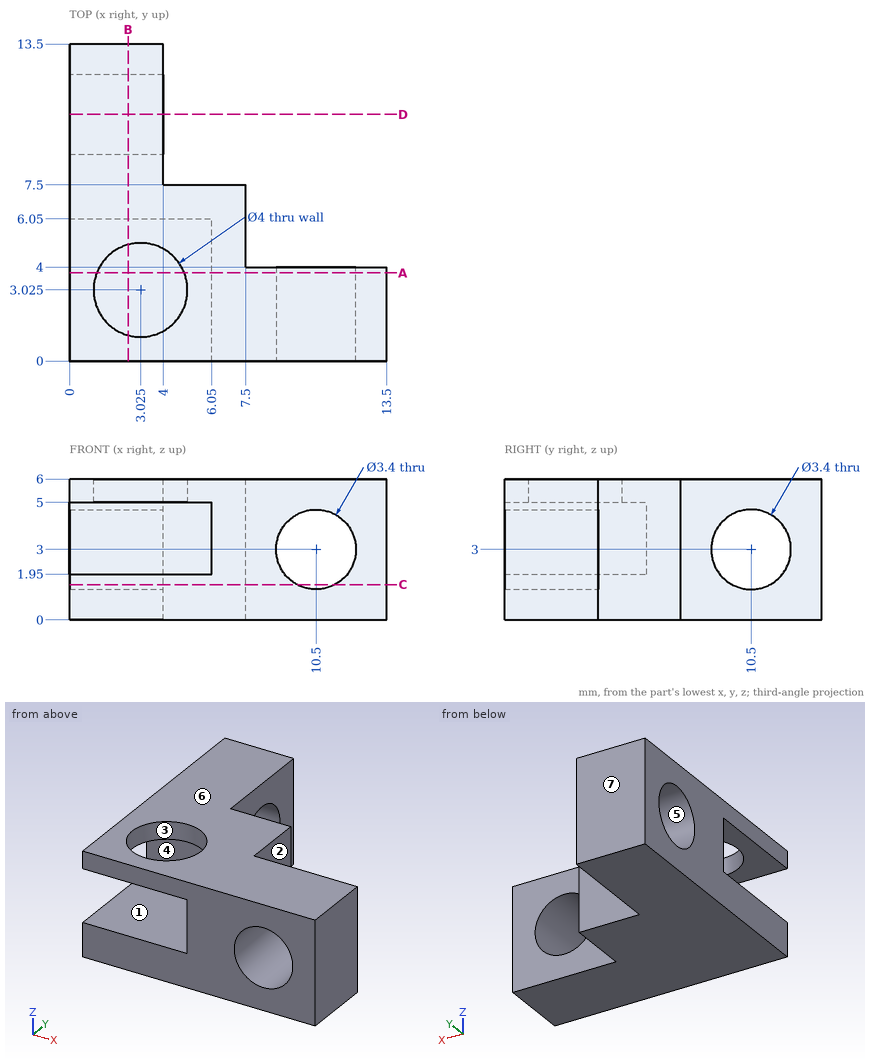
Study the drawing (mm; zero at the part's minimum x, y, z) and answer. A direction names the side the tool comes from. Round coordinates to 2 decimals unless told otherwise and drop trailing zeros. Order: outer loops, then holes, each group sorted by start corner. A loop starts at its lowest first (then second) coordinate and runs counter-clockwise, first axis right, second up. Notation, with made-up numbers: M 31,68.25 L 63,68.25 A28 cw 63,102.25 Z; hole C 76.5,-7.75 d11. An arc over 180 degrees is marked long. One line per item, written item: value.
Q1. Find section C-C on z = 1.5. Write down the section's boundary in (x, y), then the cut area to 4 significant figures.
Derived:
outline: M 0,0 L 9.7,0 L 9.7,4 L 7.5,4 L 7.5,7.5 L 4,7.5 L 4,9.7 L 0,9.7 Z; M 0,11.3 L 4,11.3 L 4,13.5 L 0,13.5 Z; M 11.3,0 L 13.5,0 L 13.5,4 L 11.3,4 Z
area: 91.45 mm²
Q2. Find section A-A on y = 3.75. Write down the section's boundary in (x, z).
Derived:
outline: M 0,0 L 13.5,0 L 13.5,6 L 4.89,6 L 4.89,5 L 6.05,5 L 6.05,1.95 L 0,1.95 Z; M 0,5 L 1.16,5 L 1.16,6 L 0,6 Z; hole C 10.5,3 d3.4
Q3. Straight lines are drawn through the part: line 1 (Z direction, x = 1.95, y = 10.5); line 2 (Y direction, x = 2.5, z = 2.9); line 3 (Z direction, x = 3, y = 2). For each, find the intervals that lie inside material, in ascending order.
Derived:
line 1: 0 to 1.3, 4.7 to 6
line 2: 6.05 to 8.8, 12.2 to 13.5
line 3: 0 to 1.95
Q4. Find section D-D on y = 10.5. Write down the section's boundary in (x, z).
Derived:
outline: M 0,0 L 4,0 L 4,1.3 L 0,1.3 Z; M 0,4.7 L 4,4.7 L 4,6 L 0,6 Z
Q5. Find section B-B on x = 2.5. Write down the section's boundary in (y, z).
Derived:
outline: M 0,0 L 13.5,0 L 13.5,6 L 4.95,6 L 4.95,5 L 6.05,5 L 6.05,1.95 L 0,1.95 Z; M 0,5 L 1.1,5 L 1.1,6 L 0,6 Z; hole C 10.5,3 d3.4
Q6. Flat-ended cylindrical pins translate along their axes: pin 1 (8 mm diameter, centred on x = 4, y = 2.5, fed in from -Z); pin 2 (0.9 mm diameter, centred on y = 4, z = 3, fed in from -X); pin 3 (3.5 mm diameter, centred on x = 3.025, y = 3.025, fed in from +Z); pin 4 (1 mm diameter, centred on y = 5, z = 2.5, fed in from +X). Find the tip coordinate at first contact, or state that the pin passes through.
Derived:
pin 1: z = 0
pin 2: x = 6.05
pin 3: z = 1.95
pin 4: x = 7.5
Q7. For the marked faces 1, 2 and 3, determine the directions among +Z, -Z, +X, -X, +Y, -Y from which every point of the face is accessible in a straight line to the end or side of a thin tool.
Derived:
face 1: -X, -Y
face 2: +Z, -Z, +X, +Y
face 3: +Z
Q8. Determine the mould class of the marked faces 4, 5, 6 and 7 for opening direction Y: released by +Y, released by -Y, zero draft, split by the parting line, or undercut.
Derived:
face 4: released by -Y
face 5: undercut
face 6: zero draft
face 7: released by +Y
